Can you work these out from the model? Positions are in its coordinate system, mm. A direction names the side the tool comes from. Coordinates: 2 decimals unless noted, no trailing zeros. Loops run counter-clockwise (first coordinate to the right, second up) from the corner with the lowest first, then second, coordinate; pieces in that order, holes last. Notation, with made-up numbers: M 28.25,48.5 L 78.25,48.5 A18 cw 78.25,77.5 Z; hole C -5.5,42.25 d3. An arc over 180 degrees is marked long. Return JSON: item names as keys, results as strings. Group by question number.
```python
from build123d import *

# Parameters (mm, degrees)
SKETCH_1_W          = 23.4
SKETCH_1_H          = 12
SKETCH_1_W_2        = 7.4
SKETCH_1_H_2        = 7
EXTRUDE_1_DEPTH     = 9.5
CUT_EXTRUDE_START   = 9.5
SKETCH_1_4_W        = 23.4
SKETCH_1_4_H        = 3
CUT_EXTRUDE_2_DEPTH = 1
SKETCH_2_W          = 19.4
SKETCH_2_H          = 8
CUT_EXTRUDE_3_DEPTH = 2


with BuildPart() as part:
    # 草图1 → 凸台-拉伸1 (new body)
    with BuildSketch(Plane(origin=(0, 0, 0), x_dir=(1, 0, 0), z_dir=(0, 1, 0))):
        with Locations((11.7, -6)):
            Rectangle(SKETCH_1_W, SKETCH_1_H)
        with Locations((12.7, -6)):
            Rectangle(SKETCH_1_W_2, SKETCH_1_H_2, mode=Mode.SUBTRACT)
    extrude(amount=EXTRUDE_1_DEPTH)

    # 草图1<4> → 切除-拉伸2 (cut)
    with BuildSketch(Plane(origin=(0, 0, 0), x_dir=(1, 0, 0), z_dir=(0, 1, 0)).offset(CUT_EXTRUDE_START)):
        with Locations((11.7, -6)):
            Rectangle(SKETCH_1_4_W, SKETCH_1_4_H)
    extrude(amount=-CUT_EXTRUDE_2_DEPTH, mode=Mode.SUBTRACT)

    # 草图2 → 切除-拉伸3 (cut)
    with BuildSketch(Plane(origin=(0, 9.5, 0), x_dir=(1, 0, 0), z_dir=(0, 1, 0))):
        with Locations((11.7, -6)):
            Rectangle(SKETCH_2_W, SKETCH_2_H)
    extrude(amount=-CUT_EXTRUDE_3_DEPTH, mode=Mode.SUBTRACT)


solid = part.part
```
1) If we mould it in two halves opening along Z, with no side actions, what happens to faces 5 (the face through (12, 9.5, 11)), 6 (the face through (12, 5, 0)), 7 (the face through (22, 9, 7.5))? For each: +Z half, -Z half, draft (parallel to the pull), parting line (faces both ways), or undercut.
2) If I drill on line 1 (X direction, y = 1.5, z = 8); line 2 (Z direction, x = 6.5, y = 8.25); line 3 (X direction, y = 7.75, z = 8.5), over which ranges is the centre line in solid material (lowest first)? Write a range as from..to.
3) Suppose I cut it at B-B, the plane x = 10. List the corners of the cut face in (y, z) for me, then the cut area to 3 significant figures.
4) For faces 1 (the face through (23.4, 5, 6)), 2 (the face through (13, 4, 9.5)), 3 (the face through (2, 8, 6)), 4 (the face through (1, 8.5, 6)), which set-ups out of +Z, -Z, +X, -X, +Y, -Y let a thin tool reach every point of the face, with its end or its side?
5) For pin 1 (1.5 mm diameter, centred on x = 13.5, z = 8.5, fed in from +Y); pin 2 (1 mm diameter, centred on x = 19, z = 5, fed in from +Y); pin 3 (1.6 mm diameter, centred on x = 22.5, z = 6.5, fed in from +Y), each with a flat end and sliding along its axis, tell me the tip position at first contact or that it passes through.
6) Suppose I cut it at C-C, the plane y = 7.75. List the corners of the cut face in (x, z) for me, then the cut area to 3 significant figures.
7) Suppose I cut it at D-D, the plane x = 5.5. List the corners of the cut face in (y, z) for me.
8) Suppose I cut it at A-A, the plane z = 5. List the corners of the cut face in (x, y) for me.
Returned:
{
 "1": {"face 5": "draft", "face 6": "-Z half", "face 7": "undercut"},
 "2": {"line 1": "x = 0..9, 16.4..23.4", "line 2": "z = 0..2, 10..12", "line 3": "x = 0..2, 21.4..23.4"},
 "3": {"outline": "M 0,0 L 9.5,0 L 9.5,2 L 7.5,2 L 7.5,2.5 L 0,2.5 Z; M 0,9.5 L 7.5,9.5 L 7.5,10 L 9.5,10 L 9.5,12 L 0,12 Z", "area": "45.5 mm²"},
 "4": {"face 1": "+Z, -Z, +X, +Y, -Y", "face 2": "+Y, -Y", "face 3": "+Y", "face 4": "+X, -X, +Y"},
 "5": {"pin 1": "passes through", "pin 2": "stops at y = 7.5", "pin 3": "stops at y = 8.5"},
 "6": {"outline": "M 0,0 L 23.4,0 L 23.4,12 L 0,12 Z; hole M 2,2 L 21.4,2 L 21.4,10 L 2,10 Z", "area": "126 mm²"},
 "7": {"outline": "M 0,0 L 9.5,0 L 9.5,2 L 7.5,2 L 7.5,10 L 9.5,10 L 9.5,12 L 0,12 Z"},
 "8": {"outline": "M 0,0 L 9,0 L 9,7.5 L 2,7.5 L 2,8.5 L 0,8.5 Z; M 16.4,0 L 23.4,0 L 23.4,8.5 L 21.4,8.5 L 21.4,7.5 L 16.4,7.5 Z"}
}
